Print and shaded views of the part. All mm, measured from the part's lowest x, y and z. A direction names the side the tool comes from. Round coordinates to 2 decimals unless told otherwise and drop trailing zeros. Order: outer loops, then holes, each group sorted by start corner. A loop starts at its lowest first (then second) coordinate and runs counter-clockwise, first axis right, second up. Notation, with made-up numbers: (84.5, 66) -> (97.5, 66) arc R19 ccw to (97.5, 93) -> close; hole circle Ø11 at (39, 34). An arc over 180 degrees is marked (long way). Answer as CSV lines item,"result". Start each with the question number.
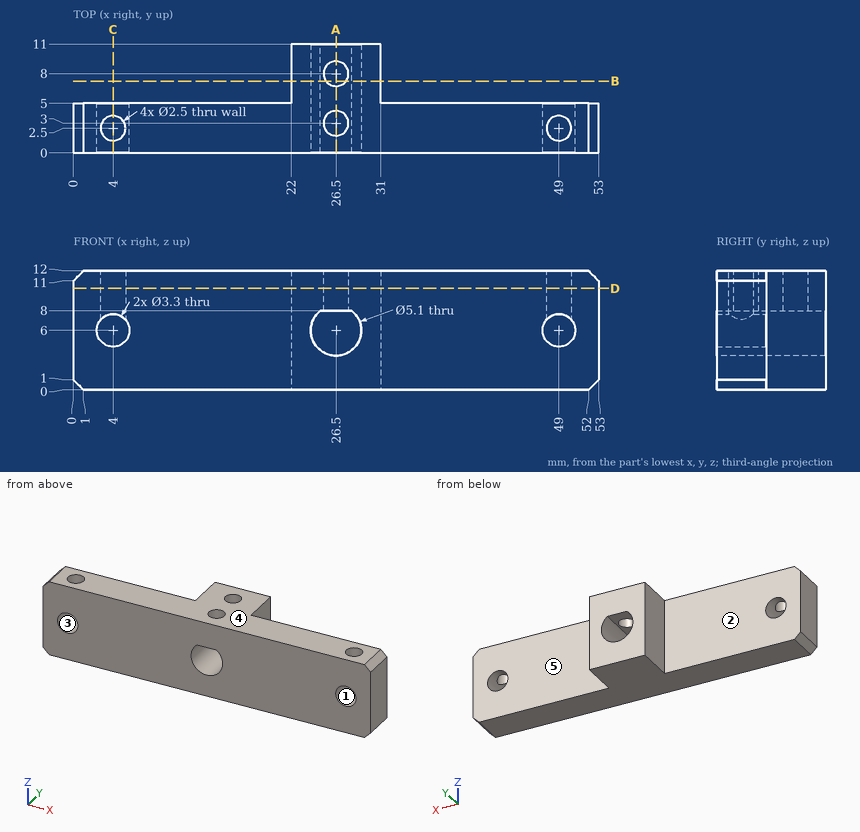
Item 1: Band-saw the part on C-C, the plane x = 4. Give the cut face in (y, z), and give its area (3 significant figures).
Item 2: Mould opens along Z. For the marked faces 3, 4 and 5 say: released by +Z, released by -Z, zero draft, split by the parting line, or undercut.
Item 3: Band-saw the part on A-A, the plane x = 26.5. Give the cut face in (y, z).
Item 4: Band-saw the part on B-B, the plane y = 7.25. Give the cut face in (x, z).
Item 5: Probe line 1 (Y direction, x = 26.5, z = 11); line 2 (X direction, y = 4.5, z = 5.25); line 3 (Y direction, x = 4, z = 8.8). List the from-to ranges inside material, lowest first.
Item 6: Pin check, flat tips, straight feed: pin 1 (6.5 mm diameter, centred on y = 7.5, z = 8.5, fed in from -X); pin 2 (1.8 mm diameter, centred on y = 7, z = 6, fed in from +X); pin 3 (3 mm diameter, centred on x = 26.5, z = 6, fed in from +Y); pin 4 (3.5 mm diameter, centred on x = 36.5, z = 3, fed in from +Y). Stop position of each tip, or through.
Item 7: Band-saw the part on D-D, the plane z = 10.25. Give the cut face in (x, y).
Item 8: Tool access for the marked faces 1 and 2: list every direction of +Z, -Z, +X, -X, +Y, -Y with a clear straight run to the whole face (end or side of a thin tool).
Values:
1,outline,"(0, 0) -> (5, 0) -> (5, 4.35) -> (0, 4.35) -> close; (0, 7.65) -> (1.25, 7.65) -> (1.25, 12) -> (0, 12) -> close; (3.75, 7.65) -> (5, 7.65) -> (5, 12) -> (3.75, 12) -> close"
1,area,"32.6 mm²"
2,face 3,"undercut"
2,face 4,"released by +Z"
2,face 5,"zero draft"
3,outline,"(0, 0) -> (11, 0) -> (11, 3.45) -> (0, 3.45) -> close; (0, 8) -> (1.75, 8) -> (1.75, 12) -> (0, 12) -> close; (4.25, 8) -> (6.75, 8) -> (6.75, 12) -> (4.25, 12) -> close; (9.25, 8) -> (11, 8) -> (11, 12) -> (9.25, 12) -> close"
4,outline,"(22, 0) -> (31, 0) -> (31, 12) -> (27.5, 12) -> (27.5, 8) -> (28.08, 8) arc R2.55 cw (long way) to (24.92, 8) -> (25.5, 8) -> (25.5, 12) -> (22, 12) -> close"
5,line 1,"0 to 1.75, 4.25 to 6.75, 9.25 to 11"
5,line 2,"0 to 2.53, 5.47 to 24.06, 28.94 to 47.53, 50.47 to 53"
5,line 3,"0 to 1.25, 3.75 to 5"
6,pin 1,"x = 0"
6,pin 2,"x = 31"
6,pin 3,"through"
6,pin 4,"y = 5"
7,outline,"(0, 0) -> (53, 0) -> (53, 5) -> (31, 5) -> (31, 11) -> (22, 11) -> (22, 5) -> (0, 5) -> close; hole circle Ø2.5 at (4, 2.5); hole circle Ø2.5 at (26.5, 3); hole circle Ø2.5 at (26.5, 8); hole circle Ø2.5 at (49, 2.5)"
8,face 1,"+Y, -Y"
8,face 2,"+Z, -Z, -X, +Y"
